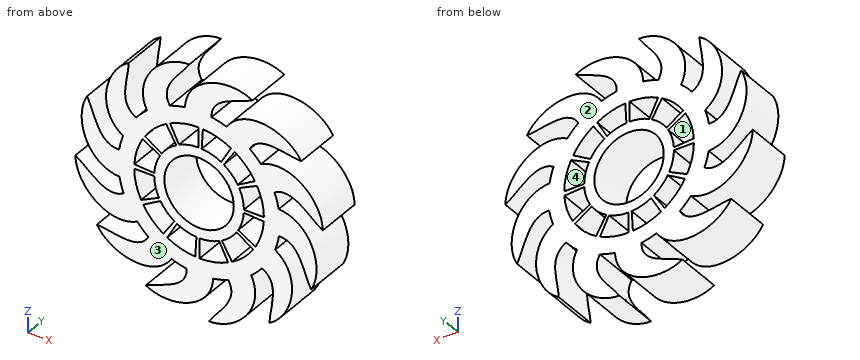
from build123d import *

# Parameters (mm, degrees)
F0_R     = 19.05
F1_DEPTH = 25.4
F3_COUNT = 12


with BuildPart() as f1:
    # F0 (on Front) → F1 (new body)
    with BuildSketch(Plane.XZ):
        with BuildLine():
            ThreePointArc((-41.7377949639, 15.1344033998), (-7.6831234343, -43.7271461338), (44.3970009653, 0))
            ThreePointArc((44.3970009653, 0), (14.7724939885, 41.8672558938), (-34.5663108784, 27.8615119291))
            ThreePointArc((-34.5663108784, 27.8615119291), (-38.6791153593, 21.7949473443), (-41.7377949639, 15.1344033998))
        make_face()
        with BuildLine():
            ThreePointArc((30.6559904103, 18.0721064124), (31.253015986, 17.0188063622), (31.8138653762, 15.9458065975))
            ThreePointArc((31.8138653762, 15.9458065975), (34.6304146039, 8.1929947261), (35.5863847309, 0))
            ThreePointArc((35.5863847309, 0), (34.4152420977, -9.0543851018), (30.9788984582, -17.5128132673))
            ThreePointArc((30.9788984582, -17.5128132673), (30.3652266448, -18.5565026077), (29.7164062853, -19.5787123096))
            ThreePointArc((29.7164062853, -19.5787123096), (17.0188063622, -31.253015986), (0.3229080478, -35.5849196797))
            ThreePointArc((0.3229080478, -35.5849196797), (-0.8877893412, -35.5753089699), (-2.0974590909, -35.5245189071))
            ThreePointArc((-2.0974590909, -35.5245189071), (-18.5565026077, -30.3652266448), (-30.6559904103, -18.0721064124))
            ThreePointArc((-30.6559904103, -18.0721064124), (-31.253015986, -17.0188063622), (-31.8138653762, -15.9458065975))
            ThreePointArc((-31.8138653762, -15.9458065975), (-35.5753089699, 0.8877893412), (-30.9788984582, 17.5128132673))
            ThreePointArc((-30.9788984582, 17.5128132673), (-30.3652266448, 18.5565026077), (-29.7164062853, 19.5787123096))
            ThreePointArc((-29.7164062853, 19.5787123096), (-17.0188063622, 31.253015986), (-0.3229080478, 35.5849196797))
            ThreePointArc((-0.3229080478, 35.5849196797), (0.8877893412, 35.5753089699), (2.0974590909, 35.5245189071))
            ThreePointArc((2.0974590909, 35.5245189071), (18.5565026077, 30.3652266448), (30.6559904103, 18.0721064124))
        make_face(mode=Mode.SUBTRACT)
        with BuildLine():
            ThreePointArc((-41.7377949639, 15.1344033998), (-38.6791153593, 21.7949473443), (-34.5663108784, 27.8615119291))
            add(Edge.make_bspline(
                [(-38.603553939, 56.0993393118), (-38.8812801549, 46.9344672316), (-44.8523311706, 33.3260222193), (-34.5663108784, 27.8615119291)],
                knots=[0, 0, 0, 0, 28.5249754922, 28.5249754922, 28.5249754922, 28.5249754922], degree=3))
            add(Edge.make_bspline(
                [(-41.7377949639, 15.1344033998), (-56.6555790407, 24.577734095), (-52.2119989513, 48.0453613593), (-38.603553939, 56.0993393118)],
                knots=[0, 0, 0, 0, 41.0846618713, 41.0846618713, 41.0846618713, 41.0846618713], degree=3))
        make_face()
        with BuildLine():
            Line((30.9788984582, -17.5128132673), (21.4377224413, -12.1190503432))
            ThreePointArc((21.4377224413, -12.1190503432), (21.0130551141, -12.8412943062), (20.5640646247, -13.5486741344))
            Line((20.5640646247, -13.5486741344), (29.7164062853, -19.5787123096))
            ThreePointArc((29.7164062853, -19.5787123096), (30.3652266448, -18.5565026077), (30.9788984582, -17.5128132673))
        make_face()
        with BuildLine():
            ThreePointArc((21.2142666876, 12.5060870618), (21.6274146437, 11.7771923869), (22.0155283003, 11.0346653029))
            Line((22.0155283003, 11.0346653029), (31.8138653762, 15.9458065975))
            ThreePointArc((31.8138653762, 15.9458065975), (31.253015986, 17.0188063622), (30.6559904103, 18.0721064124))
            Line((30.6559904103, 18.0721064124), (21.2142666876, 12.5060870618))
        make_face()
        with BuildLine():
            ThreePointArc((-0.2234557537, 24.625137405), (0.6143595296, 24.6184866931), (1.4514636756, 24.5833394373))
            Line((1.4514636756, 24.5833394373), (2.0974590909, 35.5245189071))
            ThreePointArc((2.0974590909, 35.5245189071), (0.8877893412, 35.5753089699), (-0.3229080478, 35.5849196797))
            Line((-0.3229080478, 35.5849196797), (-0.2234557537, 24.625137405))
        make_face()
        with BuildLine():
            ThreePointArc((-21.4377224413, 12.1190503432), (-21.0130551141, 12.8412943062), (-20.5640646247, 13.5486741344))
            Line((-20.5640646247, 13.5486741344), (-29.7164062853, 19.5787123096))
            ThreePointArc((-29.7164062853, 19.5787123096), (-30.3652266448, 18.5565026077), (-30.9788984582, 17.5128132673))
            Line((-30.9788984582, 17.5128132673), (-21.4377224413, 12.1190503432))
        make_face()
        with BuildLine():
            Line((-30.6559904103, -18.0721064124), (-21.2142666876, -12.5060870618))
            ThreePointArc((-21.2142666876, -12.5060870618), (-21.6274146437, -11.7771923869), (-22.0155283003, -11.0346653029))
            Line((-22.0155283003, -11.0346653029), (-31.8138653762, -15.9458065975))
            ThreePointArc((-31.8138653762, -15.9458065975), (-31.253015986, -17.0188063622), (-30.6559904103, -18.0721064124))
        make_face()
        with BuildLine():
            Line((0.3229080478, -35.5849196797), (0.2234557537, -24.625137405))
            ThreePointArc((0.2234557537, -24.625137405), (-0.6143595296, -24.6184866931), (-1.4514636756, -24.5833394373))
            Line((-1.4514636756, -24.5833394373), (-2.0974590909, -35.5245189071))
            ThreePointArc((-2.0974590909, -35.5245189071), (-0.8877893412, -35.5753089699), (0.3229080478, -35.5849196797))
        make_face()
        with BuildLine():
            ThreePointArc((21.4377224413, -12.1190503432), (23.8157082582, -6.2657293949), (24.6261512358, 0))
            ThreePointArc((24.6261512358, 0), (23.9646098878, 5.6696382261), (22.0155283003, 11.0346653029))
            ThreePointArc((22.0155283003, 11.0346653029), (21.6274146437, 11.7771923869), (21.2142666876, 12.5060870618))
            ThreePointArc((21.2142666876, 12.5060870618), (12.8412943062, 21.0130551141), (1.4514636756, 24.5833394373))
            ThreePointArc((1.4514636756, 24.5833394373), (0.6143595296, 24.6184866931), (-0.2234557537, 24.625137405))
            ThreePointArc((-0.2234557537, 24.625137405), (-11.7771923869, 21.6274146437), (-20.5640646247, 13.5486741344))
            ThreePointArc((-20.5640646247, 13.5486741344), (-21.0130551141, 12.8412943062), (-21.4377224413, 12.1190503432))
            ThreePointArc((-21.4377224413, 12.1190503432), (-24.6184866931, 0.6143595296), (-22.0155283003, -11.0346653029))
            ThreePointArc((-22.0155283003, -11.0346653029), (-21.6274146437, -11.7771923869), (-21.2142666876, -12.5060870618))
            ThreePointArc((-21.2142666876, -12.5060870618), (-12.8412943062, -21.0130551141), (-1.4514636756, -24.5833394373))
            ThreePointArc((-1.4514636756, -24.5833394373), (-0.6143595296, -24.6184866931), (0.2234557537, -24.625137405))
            ThreePointArc((0.2234557537, -24.625137405), (11.7771923869, -21.6274146437), (20.5640646247, -13.5486741344))
            ThreePointArc((20.5640646247, -13.5486741344), (21.0130551141, -12.8412943062), (21.4377224413, -12.1190503432))
        make_face()
        Circle(F0_R, mode=Mode.SUBTRACT)
    extrude(amount=F1_DEPTH)

    # F3: F1 ×12 about axis
    f3_axis = Axis((0, -7.1261581033, 0), (0, -1, 0))


with BuildPart() as f1_1:
    add(f1.part)
    for i in range(1, F3_COUNT):
        add(f1.part.rotate(f3_axis, i * 360 / F3_COUNT))


solid = f1_1.part
Model file for the job. Use its own axes, mm. Face numbers are marked on the shaded views. A direction names the side the tool comes from. Round coordinates to 2 decimals unless told otherwise and drop trailing zeros. Answer as CSV lines item,"result". Start each with the question number.
1) Slice it at A-A (y = -10.25). State how many separate pieces and enclosed holes the cut face has, plus the area to 3 significant figures.
2) Mould opens along X. For the marked faces 1 and 2 say: +X half, -X half, draft (parallel to the pull), parting line (faces both ways), or undercut.
3) Tool access for the marked faces 3 and 4: list every direction of +Z, -Z, +X, -X, +Y, -Y with a clear straight run to the whole face (end or side of a thin tool).
4) Probe line 1 along X through (y, z) = (-9.75, -44.5); line 2 along X through (y, z) = (-7, -9); line 3 along X through (y, z) = (-17.75, 52). List the from-to ranges inside material, lowest first.
5) Pin check, flat tips, straight feed: P1, Ø1.5, axis at y = -19.5, z = -12.5, coming from the +X side; P2, Ø1.5, axis at y = -6, z = -4, coming from the -X side; P3, Ø1.5, axis at y = -11.5, z = -29.5, coming from the -X side; P4, Ø10, axis at x = 23.5, z = 31, coming from the +Y side. Stop position of each tip, or through.
Filled in:
1,separate pieces,"1"
1,enclosed holes,"13"
1,area,"7,520 mm2"
2,face 1,"undercut"
2,face 2,"draft"
3,face 3,"+Z, -Z, +X, -X, -Y"
3,face 4,"+Y, -Y"
4,line 1,"x = -51.04 to -17.23, -6.84 to 7.72, 17.38 to 30.78, 40.17 to 48.56"
4,line 2,"x = -67.54 to -63, -43.48 to -34.43, -22.92 to -16.79, 16.79 to 22.92, 34.43 to 43.48, 50.86 to 63.26"
4,line 3,"x = -43.65 to -39, -28.8 to -16.66, -5.57 to 10"
5,P1,"stops at x = 64.18"
5,P2,"stops at x = -55.47"
5,P3,"stops at x = -52.11"
5,P4,"stops at y = 0"
